Source: three-view drawing plus pictorial views. Frame: mm from the lowest corner of the part. A direction names the side the tool comes from. Give positions to 0.01 mm unless a question says otherwise; leave off trailing zeros. Loops run counter-clockwise (first coordinate to the right, second up) from the corner with the lowest first, then second, coordinate; pieces in that order, holes last. Notation, with made-up numbers: (-1, 40.5) - (8, 40.5) arc R31 cw to (8, 72.5) - close; hole circle Ø7 at (-28.75, 49.25). An arc over 180 degrees is marked (long way). Answer in a Markdown table with one row per item.
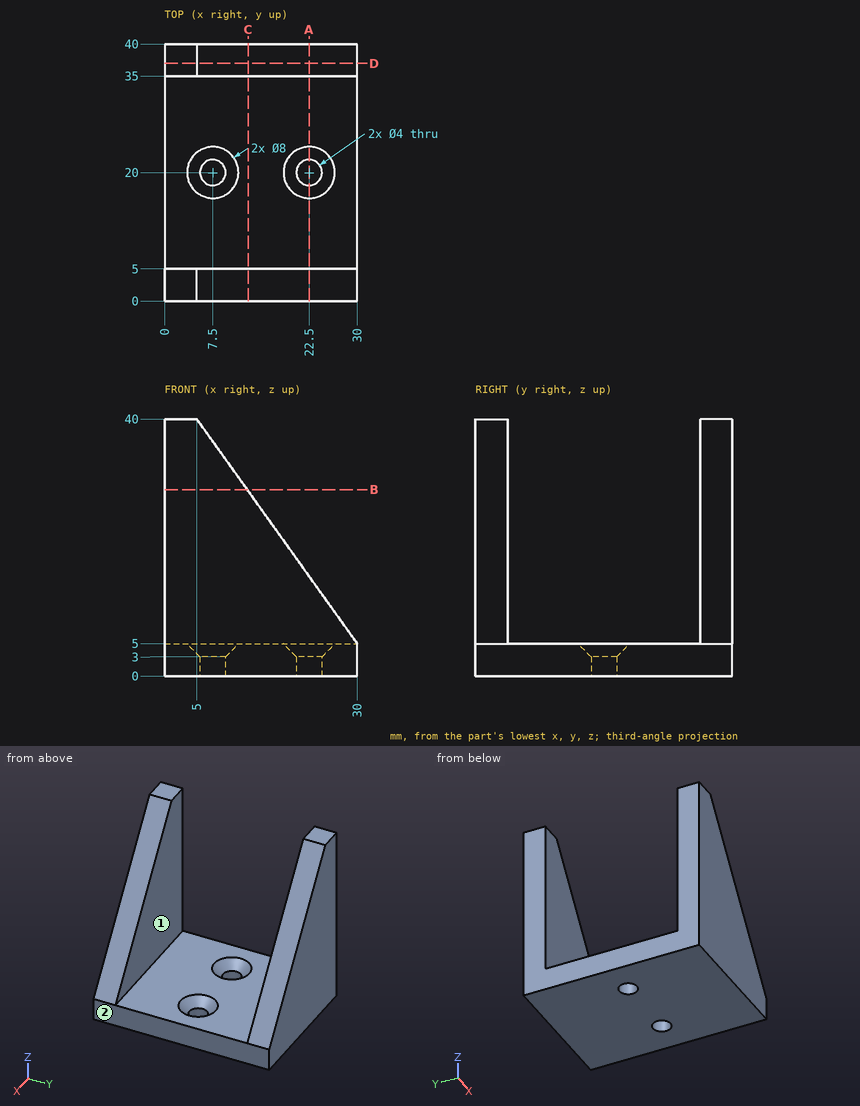
Q1. Cut plane D-D (y = 37). Output: boundary loops of the cut face in (x, z), and give its area (4 significant figures).
Check values:
| item | result |
|---|---|
| outline | (0, 0) - (30, 0) - (30, 5) - (5, 40) - (0, 40) - close |
| area | 762.5 mm² |
Q2. Reachability of the marked faces 1 and 2 from +Z, -Z, +X, -X, +Y, -Y: full face, straight path, thin tool, end or side. Return the list, or none.
Check values:
| item | result |
|---|---|
| face 1 | +Z, +X, -X |
| face 2 | +Z, -Z, +X, +Y, -Y |
Q3. Material intervals for line 1 along Y through (x, z) = (2, 24); line 2 along Y through (x, z) = (22.5, 2.05); line 3 along Z through (x, y) = (2.5, 17), sorted ascending.
Check values:
| item | result |
|---|---|
| line 1 | 0 to 5, 35 to 40 |
| line 2 | 0 to 18, 22 to 40 |
| line 3 | 0 to 5 |
Q4. First-contact query: pin 1 (3 mm diameter, centred on x = 7.5, y = 20, fed in from -Z); pin 2 (2 mm diameter, centred on x = 25, y = 25.5, fed in from +Z). Flat tips, straight axial feed; report the tip coordinate or a pass-through.
Check values:
| item | result |
|---|---|
| pin 1 | through |
| pin 2 | z = 5 |
Q5. Cut plane C-C (x = 13). Output: boundary loops of the cut face in (y, z).
Check values:
| item | result |
|---|---|
| outline | (0, 0) - (40, 0) - (40, 28.8) - (35, 28.8) - (35, 5) - (5, 5) - (5, 28.8) - (0, 28.8) - close |
Q6. Cut plane B-B (z = 29). Output: boundary loops of the cut face in (x, y).
Check values:
| item | result |
|---|---|
| outline | (0, 0) - (12.86, 0) - (12.86, 5) - (0, 5) - close; (0, 35) - (12.86, 35) - (12.86, 40) - (0, 40) - close |
Q7. Cut plane A-A (x = 22.5). Output: boundary loops of the cut face in (y, z), and give its area (3 significant figures).
Check values:
| item | result |
|---|---|
| outline | (0, 0) - (18, 0) - (18, 3) - (16, 5) - (5, 5) - (5, 15.5) - (0, 15.5) - close; (22, 0) - (40, 0) - (40, 15.5) - (35, 15.5) - (35, 5) - (24, 5) - (22, 3) - close |
| area | 281 mm² |
